Geometry check sheet. Reference: the model listing, model coordinates, mm. A direction names the side the tool comes from. Round coordinates to 2 decimals unless told otherwise and drop trailing zeros. Order: outer loops, then holes, each group sorted by start corner. A loop starts at its lowest first (then second) coordinate and runs counter-clockwise, first axis right, second up. Notation, with made-up numbers: (31.25, 46.5) -> (79.25, 46.5) arc R25 ccw to (79.25, 58.5) -> close; hole circle Ø2 at (34.5, 44.25). An arc over 180 degrees is marked (long way). Use a Markdown table: item, result. Add a question column.
Item 1: Sectioned sample at C-C, the plane y = -2. Record the cut outline in (x, z), and give its area (3 significant figures).
Item 2: Gauge pin test, flat ends, axial feed: pin 1 Ø0.6 at (y, z) = (-16.5, 1) entering from -X; pin 2 Ø0.6 at (y, z) = (17, 1) entering from -X (3 decimals). Record the tip position at first contact, or that the pin passes through.
Item 3: Mould release check, pull along X, two halves, no side actions. Record for faces 1 (the cylindrical face through (114.1, 19.14, 0.99)), 2 (the flat face through (75.37, -3.69, 0.99)), 3 (the flat face through (48, 14, 0)): pulls with the +X half, pulls with the -X half, needs draft (parallel to the pull), parting line crosses it, or undercut.
Item 4: Sectioned sample at D-D, the plane y = -10. Record the cut outline in (x, z), and give its area (3 significant figures).
Item 5: Sectioned sample at B-B, the plane z = 1.45. State how many separate pieces and enclosed holes the cut face has, and give its area (3 significant figures).
Item 6: Material ranges on probe 1 along Y at (x, z) = (30, 0.85); probe 2 along Y at (x, z) = (46.5, 0.35); probe 3 along X at (y, z) = (2.5, 0.1), recorded low to high. Write a range as [from, to].
Item 7: Set-up check for faces 4 (the cylindrical face through (15.869, -10.795, 0.986)), 5 (the flat face through (48, 14, 2)): record each of +Z, -Z, +X, -X, +Y, -Y from which the full face is reachable in a straight line by a thin tool's end or side.
Item 8: Sectioned sample at A-A, the plane x = 27. Record the cut outline in (y, z).
from build123d import *

# Parameters (mm, degrees)
SKETCH_1_R      = 5
SKETCH_1_R_2    = 1.5
SKETCH_1_W      = 4.2
SKETCH_1_H      = 2.2
EXTRUDE_1_DEPTH = 2


with BuildPart() as part:
    # 草图1 → 凸台-拉伸1 (new body)
    with BuildSketch(Plane.XY):
        with BuildLine():
            Line((0, 20), (112, 20))
            ThreePointArc((112, 20), (114.121320344, 19.121320344), (115, 17))
            Line((115, 17), (115, 8.938182396))
            ThreePointArc((115, 8.938182396), (114.544077651, 7.348317965), (113.314887395, 6.241690019))
            Line((113.314887395, 6.241690019), (60.122415269, -19.696492377))
            ThreePointArc((60.122415269, -19.696492377), (59.482258513, -19.923138479), (58.807527874, -20))
            Line((58.807527874, -20), (0, -20))
            ThreePointArc((0, -20), (-20, 0), (0, 20))
        make_face()
        Circle(SKETCH_1_R, mode=Mode.SUBTRACT)
        with Locations(Location((30, 16.9, 0), (0, 0, 180))):
            Circle(SKETCH_1_R_2, mode=Mode.SUBTRACT)
        with Locations(Location((105.6, 16.9, 0), (0, 0, 180))):
            Circle(SKETCH_1_R_2, mode=Mode.SUBTRACT)
        with Locations((59.5, -16.9)):
            Circle(SKETCH_1_R_2, mode=Mode.SUBTRACT)
        with BuildLine():
            Line((59.567545449, -11.393906383), (91.618526066, 4.235075463))
            ThreePointArc((91.618526066, 4.235075463), (93.22677715, 7.606298478), (90.303638671, 9.93156784))
            Line((90.303638671, 9.93156784), (18.013127748, 9.93156784))
            ThreePointArc((18.013127748, 9.93156784), (15.891807404, 9.052888183), (15.013127748, 6.93156784))
            Line((15.013127748, 6.93156784), (15.013127748, -8.697414007))
            ThreePointArc((15.013127748, -8.697414007), (15.891807404, -10.81873435), (18.013127748, -11.697414007))
            Line((18.013127748, -11.697414007), (58.252658054, -11.697414007))
            ThreePointArc((58.252658054, -11.697414007), (58.927388693, -11.620552485), (59.567545449, -11.393906383))
        make_face(mode=Mode.SUBTRACT)
        with Locations((99.6, 16.9)):
            Rectangle(SKETCH_1_W, SKETCH_1_H, mode=Mode.SUBTRACT)
        with Locations((36, 16.9)):
            Rectangle(SKETCH_1_W, SKETCH_1_H, mode=Mode.SUBTRACT)
        with Locations((53.5, -16.9)):
            Rectangle(SKETCH_1_W, SKETCH_1_H, mode=Mode.SUBTRACT)
    extrude(amount=EXTRUDE_1_DEPTH)


solid = part.part
Found:
| question | item | result |
|---|---|---|
| 1 | outline | (-19.9, 0) -> (-4.58, 0) -> (-4.58, 2) -> (-19.9, 2) -> close; (4.58, 0) -> (15.01, 0) -> (15.01, 2) -> (4.58, 2) -> close; (78.83, 0) -> (96.41, 0) -> (96.41, 2) -> (78.83, 2) -> close |
| 1 | area | 86.7 mm2 |
| 2 | pin 1 | stops at x = -11.73 |
| 2 | pin 2 | stops at x = -11.005 |
| 3 | face 1 | pulls with the +X half |
| 3 | face 2 | undercut |
| 3 | face 3 | needs draft |
| 4 | outline | (-17.32, 0) -> (15.31, 0) -> (15.31, 2) -> (-17.32, 2) -> close; (62.43, 0) -> (80.01, 0) -> (80.01, 2) -> (62.43, 2) -> close |
| 4 | area | 100 mm2 |
| 5 | separate pieces | 1 |
| 5 | enclosed holes | 8 |
| 5 | area | 2,950 mm2 |
| 6 | probe 1 | y = [-20, -11.7], [9.93, 15.4], [18.4, 20] |
| 6 | probe 2 | y = [-20, -11.7], [9.93, 20] |
| 6 | probe 3 | x = [-19.84, -4.33], [4.33, 15.01], [88.06, 105.64] |
| 7 | face 4 | +Z, -Z |
| 7 | face 5 | +Z, +X, -X, +Y, -Y |
| 8 | outline | (-20, 0) -> (-11.7, 0) -> (-11.7, 2) -> (-20, 2) -> close; (9.93, 0) -> (20, 0) -> (20, 2) -> (9.93, 2) -> close |
